Could you check a few things on this model? Use its own coordinates, in mm. A direction names the side the tool comes from. Give positions to 0.01 mm unless a question says otherwise; leave off trailing zeros. Loops run counter-clockwise (first coordinate to the right, second up) from the corner with the lowest first, then second, coordinate; pieces in that order, holes last. Notation, with made-up numbers: (47.5, 67) -> (56.5, 67) arc R21 cw to (56.5, 81) -> close; hole circle Ø2 at (59.5, -29). An arc over 180 degrees is marked (long way). Put each result on its own line as item: value.
```python
from build123d import *

# Parameters (mm, degrees)
SKETCH_1_W          = 165
SKETCH_1_H          = 100
EXTRUDE_1_DEPTH     = 3.5
SKETCH_2_W          = 35
SKETCH_2_H          = 12
SKETCH_2_W_2        = 5
SKETCH_2_H_2        = 80
SKETCH_2_W_3        = 30
EXTRUDE_2_DEPTH     = 2
EXTRUDE_3_DEPTH     = 1.5
SKETCH_4_W          = 90
SKETCH_4_H          = 64
EXTRUDE_4_DEPTH     = 1.5
SKETCH_5_R          = 1.5
EXTRUDE_5_DEPTH     = 7
SKETCH_6_W          = 90
SKETCH_6_H          = 64
SKETCH_6_W_2        = 6.8
SKETCH_6_H_2        = 16
SKETCH_6_H_3        = 10.5
SKETCH_6_H_4        = 8.5
SKETCH_6_W_3        = 5
SKETCH_6_H_5        = 2.5
EXTRUDE_6_DEPTH     = 1.5
SKETCH_7_R          = 1.5
EXTRUDE_7_DEPTH     = 7
SKETCH_8_W          = 157
SKETCH_8_H          = 89
CUT_EXTRUDE_1_DEPTH = 0.1


with BuildPart() as part:
    # 草图1 → 凸台-拉伸1 (new body)
    with BuildSketch(Plane(origin=(0, 0, 0), x_dir=(1, 0, 0), z_dir=(0, 1, 0))):
        Rectangle(SKETCH_1_W, SKETCH_1_H)
    extrude(amount=EXTRUDE_1_DEPTH)

    # 草图2 → 凸台-拉伸2 (add)
    with BuildSketch(Plane.XZ):
        with Locations((0, 39)):
            Rectangle(SKETCH_2_W, SKETCH_2_H)
        with Locations((-75, 0)):
            Rectangle(SKETCH_2_W_2, SKETCH_2_H_2)
        with Locations((75, 0)):
            Rectangle(SKETCH_2_W_2, SKETCH_2_H_2)
        with Locations((-42.5, -39)):
            Rectangle(SKETCH_2_W_3, SKETCH_2_H)
    extrude(amount=EXTRUDE_2_DEPTH)

    # 草图3 → 凸台-拉伸3 (add)
    with BuildSketch(Plane.XZ.offset(2)):
        with BuildLine():
            Line((82.5, -54.5), (77, -54.5))
            ThreePointArc((77, -54.5), (73.5, -58), (70, -54.5))
            Line((70, -54.5), (-70, -54.5))
            ThreePointArc((-70, -54.5), (-73.5, -58), (-77, -54.5))
            Line((-77, -54.5), (-82.5, -54.5))
            Line((-82.5, -54.5), (-82.5, 51.5))
            Line((-82.5, 51.5), (82.5, 51.5))
            Line((82.5, 51.5), (82.5, -54.5))
        make_face()
    extrude(amount=EXTRUDE_3_DEPTH)

    # 草图4 → 凸台-拉伸4 (add)
    with BuildSketch(Plane.XZ.offset(3.5)):
        with Locations((0, 19.5)):
            Rectangle(SKETCH_4_W, SKETCH_4_H)
    extrude(amount=EXTRUDE_4_DEPTH)

    # 草图5 → 凸台-拉伸5 (add)
    with BuildSketch(Plane.XZ.offset(5)):
        Polygon((-33.643226867, 46.5), (-30.929680602, 46.5), (-29.57290747, 44.15), (-30.929680602, 41.8), (-33.643226867, 41.8), (-35, 44.15), align=None)
        with Locations((-32.286453735, 44.15)):
            Circle(SKETCH_5_R, mode=Mode.SUBTRACT)
        Polygon((35, 44.15), (36.356773133, 46.5), (39.070319398, 46.5), (40.42709253, 44.15), (39.070319398, 41.8), (36.356773133, 41.8), align=None)
        with Locations((37.713546265, 44.15)):
            Circle(SKETCH_5_R, mode=Mode.SUBTRACT)
        Polygon((36.356773133, -2.8), (35, -5.15), (36.356773133, -7.5), (39.070319398, -7.5), (40.42709253, -5.15), (39.070319398, -2.8), align=None)
        with Locations((37.713546265, -5.15)):
            Circle(SKETCH_5_R, mode=Mode.SUBTRACT)
        Polygon((-33.643226867, -2.8), (-35, -5.15), (-33.643226867, -7.5), (-30.929680602, -7.5), (-29.57290747, -5.15), (-30.929680602, -2.8), align=None)
        with Locations((-32.286453735, -5.15)):
            Circle(SKETCH_5_R, mode=Mode.SUBTRACT)
    extrude(amount=EXTRUDE_5_DEPTH)

    # 草图6 → 凸台-拉伸6 (add)
    with BuildSketch(Plane.XZ.offset(12)):
        with Locations((0, 19.5)):
            Rectangle(SKETCH_6_W, SKETCH_6_H)
        with Locations((-39.1, 35.5)):
            Rectangle(SKETCH_6_W_2, SKETCH_6_H_2, mode=Mode.SUBTRACT)
        with Locations((-39.1, 19.25)):
            Rectangle(SKETCH_6_W_2, SKETCH_6_H_3, mode=Mode.SUBTRACT)
        with Locations((-39.1, 6.25)):
            Rectangle(SKETCH_6_W_2, SKETCH_6_H_3, mode=Mode.SUBTRACT)
        with Locations((-39.1, -5.25)):
            Rectangle(SKETCH_6_W_2, SKETCH_6_H_4, mode=Mode.SUBTRACT)
        with Locations((31.412593709, 19.5)):
            Rectangle(SKETCH_6_W_3, SKETCH_6_H_5, mode=Mode.SUBTRACT)
    extrude(amount=EXTRUDE_6_DEPTH)

    # 草图7 → 凸台-拉伸7 (add)
    with BuildSketch(Plane.XZ.offset(3.5)):
        Polygon((-77.356773133, 47.35), (-74.643226867, 47.35), (-73.286453735, 45), (-74.643226867, 42.65), (-77.356773133, 42.65), (-78.713546265, 45), align=None)
        with Locations((-76, 45)):
            Circle(SKETCH_7_R, mode=Mode.SUBTRACT)
        Polygon((73.286453735, 45), (74.643226867, 47.35), (77.356773133, 47.35), (78.713546265, 45), (77.356773133, 42.65), (74.643226867, 42.65), align=None)
        with Locations((76, 45)):
            Circle(SKETCH_7_R, mode=Mode.SUBTRACT)
        Polygon((74.643226867, -45.65), (73.286453735, -48), (74.643226867, -50.35), (77.356773133, -50.35), (78.713546265, -48), (77.356773133, -45.65), align=None)
        with Locations((76, -48)):
            Circle(SKETCH_7_R, mode=Mode.SUBTRACT)
        Polygon((-77.356773133, -45.65), (-78.713546265, -48), (-77.356773133, -50.35), (-74.643226867, -50.35), (-73.286453735, -48), (-74.643226867, -45.65), align=None)
        with Locations((-76, -48)):
            Circle(SKETCH_7_R, mode=Mode.SUBTRACT)
    extrude(amount=EXTRUDE_7_DEPTH)

    # 草图8 → 切除-拉伸1 (cut)
    with BuildSketch(Plane(origin=(0, 3.5, 0), x_dir=(1, 0, 0), z_dir=(0, 1, 0))):
        with Locations((1.5, -2)):
            Rectangle(SKETCH_8_W, SKETCH_8_H)
    extrude(amount=-CUT_EXTRUDE_1_DEPTH, mode=Mode.SUBTRACT)


solid = part.part
```
1. If we section it at B-B (z = 7): Count the separate pieces of the cut face and the enclosed holes in it, then the cut area to 3 significant figures.
Recorded:
separate pieces: 3
enclosed holes: 1
area: 1,090 mm^2
2. I'm going to push flat-ended pins straight in: pin 1 (2.5 mm diameter, centred on x = -32.29, z = -5.15, fed in from +Y); pin 2 (0.6 mm diameter, centred on y = -1.5, z = 39.5, fed in from +X); pin 3 (1.6 mm diameter, centred on x = -76, y = -0.5, fed in from -Z); pin 4 (10 mm diameter, centred on x = -8.5, y = -10, fed in from +Z). Where does each tip first touch, or does it pass through?
Recorded:
pin 1: stops at y = 3.4
pin 2: stops at x = 77.5
pin 3: stops at z = -50
pin 4: stops at z = 51.5
3. If we section it at D-D (z = -17): List the corners of the cut face in (x, y) for me.
Recorded:
outline: (-82.5, -3.5) -> (82.5, -3.5) -> (82.5, -2) -> (77.5, -2) -> (77.5, 0) -> (82.5, 0) -> (82.5, 3.5) -> (80, 3.5) -> (80, 3.4) -> (-77, 3.4) -> (-77, 3.5) -> (-82.5, 3.5) -> (-82.5, 0) -> (-77.5, 0) -> (-77.5, -2) -> (-82.5, -2) -> close; hole (-72.5, -2) -> (72.5, -2) -> (72.5, 0) -> (-72.5, 0) -> close
4. For faces 1 (the face through (76, -10.5, -50)), 2 (the face through (36.215, -8.451, -5.084)), 3 (the face through (-75.31, -6.95, -49.33)), 4 (the face through (-1, 2, -50)), 5 (the face through (82.5, 2, 1)), which set-ups out of +Z, -Z, +X, -X, +Y, -Y let a thin tool reach every point of the face, with its end or its side?
Recorded:
face 1: +Z, -Z, +X, -X, -Y
face 2: none
face 3: -Y
face 4: -Z, +X, -X, +Y
face 5: +Z, -Z, +X, +Y, -Y
5. If we section it at A-A (x = 49): List the corners of the cut face in (y, z) for me.
Recorded:
outline: (-3.5, -54.5) -> (-2, -54.5) -> (-2, 51.5) -> (-3.5, 51.5) -> close; (0, -50) -> (3.5, -50) -> (3.5, -42.5) -> (3.4, -42.5) -> (3.4, 46.5) -> (3.5, 46.5) -> (3.5, 50) -> (0, 50) -> close
6. Thinking about a two-plate mould opening in Z: for faces 6 (the face through (-76, -3.5, -48)), 7 (the face through (73.6, -2.7, -58)), which applies, pulls with the +Z half, pulls with the -Z half, needs draft (parallel to the pull), parting line crosses it, or undercut?
Recorded:
face 6: undercut
face 7: pulls with the -Z half
7. I need wall thicknesses on line 1 (Y direction, x = 26.5, z = -6); line 2 (Z direction, x = 76, y = -5.5); line 3 (Y direction, x = -28, z = -28.5). Which ranges of each line are inside material? Lowest first, please.
Recorded:
line 1: y = -13.5 to -12, -5 to -2, 0 to 3.4
line 2: z = -50.35 to -49.5, -46.5 to -45.65, 42.65 to 43.5, 46.5 to 47.35
line 3: y = -3.5 to -2, 0 to 3.4
